Part model, mm, in its own coordinate system. Round coordinates to 2 decimals unless told otherwise and drop trailing zeros. Loops run counter-clockwise (first coordinate to the right, second up) from the corner with the lowest first, then second, coordinate; pieces in that order, holes last. Notation, with made-up numbers: (-19, -39.75) -> (-2, -39.75) arc R26 ccw to (-2, -10.75) -> close; hole circle Ø8 at (-14.75, 59). An arc over 180 degrees is marked (long way). Use a Markdown table: item, result. Add a question column.
Item 1: Flat gauge pins, fed straight in: pin 1 (10 mm diameter, centred on x = 92.5, z = -99.5, fed in from +Y); pin 2 (4.5 mm diameter, centred on x = 26.3, y = 21.36, fed in from -Z); pin 3 (0.7 mm diameter, centred on y = 25, z = -126.5, fed in from +X); pin 4 (10 mm diameter, centred on x = 86.5, y = 19, fed in from -Z). Where does each tip first touch, or does it go through?
Item 2: Cut at C-C, the plane x = 58. List the corners of the cut face in (y, z), plus the area to 3 significant figures.
Item 3: Cut at B-B, the plane z = -23.5. List the corners of the cut face in (x, y), plus the area to 3 significant figures.
Item 4: Cut at A-A, the plane x = 93.5. List the corners of the cut face in (y, z), plus the area to 3 significant figures.
Item 5: Probe line 1 (Y direction, x = -17, z = 52); line 2 (X direction, y = 21, z = -125.5). List the from-to ranges inside material, lowest first. Write a range as [from, to].
Item 6: Cut at D-D, the plane x = 9. List the corners of the cut face in (y, z), plus the area to 3 significant figures.
```python
from build123d import *

# Parameters (mm, degrees)
BOSS_EXTRUDE1_DEPTH = 6.35
SKETCH2_W           = 7.5438
SKETCH2_H           = 7.62
BOSS_EXTRUDE2_DEPTH = 19.9898
FILLET1_R           = 17.78
SKETCH3_R           = 1.3462
CUT_EXTRUDE1_DEPTH  = 5.4102


with BuildPart() as part:
    # Sketch1 → Boss-Extrude1 (new body)
    with BuildSketch(Plane(origin=(0, 0, 0), x_dir=(1, 0, 0), z_dir=(0, 1, 0))):
        with BuildLine():
            Line((88.9, 141.121005256), (50.8, 141.121005256))
            Line((50.8, 141.121005256), (50.8, -76.2))
            Line((50.8, -76.2), (103.023285942, -76.2))
            ThreePointArc((103.023285942, -76.2), (109.991730457, -74.117475267), (114.674827247, -68.552878903))
            Line((114.674827247, -68.552878903), (127, -40.132))
            Line((127, -40.132), (127, 99.568))
            Line((127, 99.568), (98.981931967, 136.144))
            ThreePointArc((98.981931967, 136.144), (94.521742023, 139.808982101), (88.9, 141.121005256))
        make_face()
        with BuildLine():
            Line((50.8, 141.121005256), (12.7, 141.121005256))
            ThreePointArc((12.7, 141.121005256), (7.078257977, 139.808982101), (2.618068033, 136.144))
            Line((2.618068033, 136.144), (-25.4, 99.568))
            Line((-25.4, 99.568), (-25.4, -40.132))
            Line((-25.4, -40.132), (-13.074827247, -68.552878903))
            ThreePointArc((-13.074827247, -68.552878903), (-8.391730457, -74.117475267), (-1.423285942, -76.2))
            Line((-1.423285942, -76.2), (50.8, -76.2))
            Line((50.8, -76.2), (50.8, 141.121005256))
        make_face()
    extrude(amount=BOSS_EXTRUDE1_DEPTH)

    # Sketch2 → Boss-Extrude2 (add)
    with BuildSketch(Plane(origin=(0, 6.35, 0), x_dir=(1, 0, 0), z_dir=(0, 1, 0))):
        with Locations((74.7268, 127.151005256)):
            Rectangle(SKETCH2_W, SKETCH2_H)
        with Locations((26.8732, 127.151005256)):
            Rectangle(SKETCH2_W, SKETCH2_H)
    extrude(amount=BOSS_EXTRUDE2_DEPTH)

    # Fillet1
    fillet1_edges = [part.edges().sort_by_distance(p)[0] for p in [
        (23.1013, 6.35, -127.151005256),
        (26.8732, 6.35, -123.341005256),
        (78.4987, 6.35, -127.151005256),
        (74.7268, 6.35, -123.341005256),
    ]]
    fillet(fillet1_edges, radius=FILLET1_R)

    # Sketch3 → Cut-Extrude1 (cut)
    with BuildSketch(Plane(origin=(0, 0, -130.961005256), x_dir=(-1, 0, 0), z_dir=(0, 0, -1))):
        with Locations((-75.2983, 11.3538)):
            Circle(SKETCH3_R)
        with Locations((-75.2983, 21.3614)):
            Circle(SKETCH3_R)
        with Locations(Location((-26.3017, 11.3538, 0), (0, 0, 180))):
            Circle(SKETCH3_R)
        with Locations(Location((-26.3017, 21.3614, 0), (0, 0, 180))):
            Circle(SKETCH3_R)
    extrude(amount=-CUT_EXTRUDE1_DEPTH, mode=Mode.SUBTRACT)


solid = part.part
```
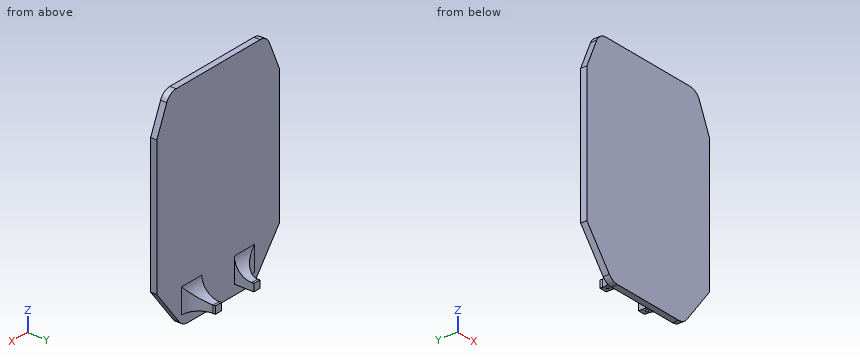
A:
| question | item | result |
|---|---|---|
| 1 | pin 1 | stops at y = 6.35 |
| 1 | pin 2 | stops at z = -130.96 |
| 1 | pin 3 | stops at x = 78.5 |
| 1 | pin 4 | passes through |
| 2 | outline | (0, -141.12) -> (6.35, -141.12) -> (6.35, 76.2) -> (0, 76.2) -> close |
| 2 | area | 1,380 mm^2 |
| 3 | outline | (-25.4, 0) -> (127, 0) -> (127, 6.35) -> (-25.4, 6.35) -> close |
| 3 | area | 968 mm^2 |
| 4 | outline | (0, -140.26) -> (6.35, -140.26) -> (6.35, -130.96) -> (6.57, -130.96) -> (6.57, -108.34) arc R17.78 cw to (6.35, -105.56) -> (6.35, 76.2) -> (0, 76.2) -> close |
| 4 | area | 1,380 mm^2 |
| 5 | line 1 | y = [0, 6.35] |
| 5 | line 2 | x = [22.82, 30.65], [70.95, 78.78] |
| 6 | outline | (0, -140.57) -> (6.35, -140.57) -> (6.35, -130.96) -> (6.73, -130.96) -> (6.73, -109.24) arc R17.78 cw to (6.35, -105.56) -> (6.35, 76.2) -> (0, 76.2) -> close |
| 6 | area | 1,390 mm^2 |
